from build123d import *

# Parameters (mm, degrees)
SKETCH_1_R          = 30
SKETCH_1_R_2        = 23
EXTRUDE_1_DEPTH     = 21
SKETCH_2_R          = 23
SKETCH_2_R_2        = 4.1
SKETCH_2_R_3        = 1.55
EXTRUDE_2_DEPTH     = 1
SKETCH_3_R          = 30
SKETCH_3_R_2        = 1.55
SKETCH_3_R_3        = 4.1
EXTRUDE_3_DEPTH     = 3
SKETCH_4_R          = 30
CUT_EXTRUDE_1_DEPTH = 3


with BuildPart() as part:
    # 草图1 → 凸台-拉伸1 (new body)
    with BuildSketch(Plane(origin=(0, 0, 0), x_dir=(1, 0, 0), z_dir=(0, 1, 0))):
        Circle(SKETCH_1_R)
        Circle(SKETCH_1_R_2, mode=Mode.SUBTRACT)
    extrude(amount=EXTRUDE_1_DEPTH)

    # 草图2 → 凸台-拉伸2 (add)
    with BuildSketch(Plane.XZ):
        Circle(SKETCH_2_R)
        Circle(SKETCH_2_R_2, mode=Mode.SUBTRACT)
        with Locations((6, 0)):
            Circle(SKETCH_2_R_3, mode=Mode.SUBTRACT)
        with Locations((-6, 0)):
            Circle(SKETCH_2_R_3, mode=Mode.SUBTRACT)
        with Locations((0, 6.5)):
            Circle(SKETCH_2_R_3, mode=Mode.SUBTRACT)
        with Locations((0, -6.5)):
            Circle(SKETCH_2_R_3, mode=Mode.SUBTRACT)
        with BuildLine():
            ThreePointArc((13.744660155, 13.324975875), (0.2967616, 19.141123201), (-13.324975875, 13.744660155))
            ThreePointArc((-13.324975875, 13.744660155), (-13.412668503, 8.088485652), (-7.756494001, 8.000793024))
            ThreePointArc((-7.756494001, 8.000793024), (0.172745496, 11.142084508), (8.000793024, 7.756494001))
            ThreePointArc((8.000793024, 7.756494001), (13.656967527, 7.668801373), (13.744660155, 13.324975875))
        make_face(mode=Mode.SUBTRACT)
        with BuildLine():
            ThreePointArc((13.744660155, -13.324975875), (0.2967616, -19.141123201), (-13.324975875, -13.744660155))
            ThreePointArc((-13.324975875, -13.744660155), (-13.412668503, -8.088485652), (-7.756494001, -8.000793024))
            ThreePointArc((-7.756494001, -8.000793024), (0.172745496, -11.142084508), (8.000793024, -7.756494001))
            ThreePointArc((8.000793024, -7.756494001), (13.656967527, -7.668801373), (13.744660155, -13.324975875))
        make_face(mode=Mode.SUBTRACT)
    extrude(amount=-EXTRUDE_2_DEPTH)

    # 草图3 → 凸台-拉伸3 (add)
    with BuildSketch(Plane.XZ):
        Circle(SKETCH_3_R)
        with Locations((0, -6.5)):
            Circle(SKETCH_3_R_2, mode=Mode.SUBTRACT)
        with Locations((6, 0)):
            Circle(SKETCH_3_R_2, mode=Mode.SUBTRACT)
        Circle(SKETCH_3_R_3, mode=Mode.SUBTRACT)
        with Locations((0, 6.5)):
            Circle(SKETCH_3_R_2, mode=Mode.SUBTRACT)
        with BuildLine():
            ThreePointArc((-7.756494001, -8.000793024), (-13.412668503, -8.088485652), (-13.324975875, -13.744660155))
            ThreePointArc((-13.324975875, -13.744660155), (0.2967616, -19.141123201), (13.744660155, -13.324975875))
            ThreePointArc((13.744660155, -13.324975875), (13.656967527, -7.668801373), (8.000793024, -7.756494001))
            ThreePointArc((8.000793024, -7.756494001), (0.172745496, -11.142084508), (-7.756494001, -8.000793024))
        make_face(mode=Mode.SUBTRACT)
        with BuildLine():
            ThreePointArc((8.000793024, 7.756494001), (13.656967527, 7.668801373), (13.744660155, 13.324975875))
            ThreePointArc((13.744660155, 13.324975875), (0.2967616, 19.141123201), (-13.324975875, 13.744660155))
            ThreePointArc((-13.324975875, 13.744660155), (-13.412668503, 8.088485652), (-7.756494001, 8.000793024))
            ThreePointArc((-7.756494001, 8.000793024), (0.172745496, 11.142084508), (8.000793024, 7.756494001))
        make_face(mode=Mode.SUBTRACT)
    extrude(amount=EXTRUDE_3_DEPTH)

    # 草图4 → 切除-拉伸1 (cut)
    with BuildSketch(Plane(origin=(0, 21, 0), x_dir=(1, 0, 0), z_dir=(0, 1, 0))):
        Circle(SKETCH_4_R)
    extrude(amount=-CUT_EXTRUDE_1_DEPTH, mode=Mode.SUBTRACT)


solid = part.part
Source: CAD feature listing. Evaluate the final solid. Frame: model axes, mm. A direction names the side the tool comes from. Coordinates: 2 decimals unless noted, no trailing zeros. Order: outer loops, then holes, each group sorted by start corner. A loop starts at its lowest first (then second) coordinate and runs counter-clockwise, first axis right, second up.
Item 1: Cut plane B-B (z = 0). Return loops of the section in (x, y), plus the area to 3 significant figures.
Output values:
outline: (-30, -3) - (-4.1, -3) - (-4.1, 1) - (-4.45, 1) - (-4.45, 0) - (-7.55, 0) - (-7.55, 1) - (-23, 1) - (-23, 18) - (-30, 18) - close; (4.1, -3) - (4.45, -3) - (4.45, 1) - (4.1, 1) - close; (7.55, -3) - (30, -3) - (30, 18) - (23, 18) - (23, 1) - (7.55, 1) - close
area: 430 mm2
Item 2: Cut plane A-A (x = 0). Return loops of the section in (y, z), plus the area to 3 significant figures.
Output values:
outline: (-3, -30) - (18, -30) - (18, -23) - (1, -23) - (1, -19.14) - (-3, -19.14) - close; (-3, -11.14) - (1, -11.14) - (1, -8.05) - (-3, -8.05) - close; (-3, -4.95) - (1, -4.95) - (1, -4.1) - (-3, -4.1) - close; (-3, 4.1) - (1, 4.1) - (1, 4.95) - (-3, 4.95) - close; (-3, 8.05) - (1, 8.05) - (1, 11.14) - (-3, 11.14) - close; (-3, 19.14) - (1, 19.14) - (1, 23) - (18, 23) - (18, 30) - (-3, 30) - close
area: 356 mm2
Item 3: Pull-direction query (Z, two-part tool) for faces 4 (the face through (-29.97, 7.65, 1.32)), 5 (the face through (-7, -3, 0)), 6 (the face through (-7.55, 0.49, 0.07)), 7 (the face through (0.3, -0.97, -11.14)); classes: pulls with the +Z half, pulls with the -Z half, needs draft (parallel to the pull), parting line crosses it, or undercut.
Output values:
face 4: parting line crosses it
face 5: needs draft
face 6: undercut
face 7: undercut
Item 4: Set-up query: faces 1 (the face through (-0.3, 1, -4.8)), 2 (the face through (0.086, -0.972, -19.143)), 3 (the face through (15, 18, 18)). Return all of +Z, -Z, +X, -X, +Y, -Y with unobstructed straight access to the full face (end or side cutting, diameter ignored); none if empty.
Output values:
face 1: +Y
face 2: +Y, -Y
face 3: +Z, -Z, +X, -X, +Y
Item 5: Material intervals for line 1 (Z direction, x = 0, y = -1.45); line 2 (Z direction, x = -6, y = 0.35); line 3 (Y direction, x = -17, z = 12), sorted ascending.
Output values:
line 1: z = -30 to -19.14, -11.14 to -8.05, -4.95 to -4.1, 4.1 to 4.95, 8.05 to 11.14, 19.14 to 30
line 2: z = -29.39 to -18.18, -9.39 to -1.55, 1.55 to 9.39, 18.18 to 29.39
line 3: y = -3 to 1
Item 6: First-contact query: P1, Ø1.5, axis at x = -5.5, z = 0.5, coming from the +Y side; P2, Ø23, axis at x = -10, z = -5.5, coming from the +Y side; P3, Ø10.5, axis at x = 0, z = 0, coming from the -Y side; P4, Ø1, axis at x = -16.5, y = 9.5, coming from the +Z side. Flat tips, straight axial feed; report the tip coordinate or a pass-through.
Output values:
P1: stops at y = 0
P2: stops at y = 1
P3: stops at y = -3
P4: stops at z = 25.38
Item 7: Cut plane D-D (y = 2.5). Return loops of the section in (x, z).
Output values:
outline: circle Ø60 at (0, 0); hole circle Ø46 at (0, 0)
Item 8: Cut plane C-C (x = -6). Return loops of the section in (y, z).
Output values:
outline: (-3, -29.39) - (18, -29.39) - (18, -22.2) - (1, -22.2) - (1, -18.18) - (-3, -18.18) - close; (-3, -9.39) - (1, -9.39) - (1, -1.55) - (0, -1.55) - (0, 1.55) - (1, 1.55) - (1, 9.39) - (-3, 9.39) - close; (-3, 18.18) - (1, 18.18) - (1, 22.2) - (18, 22.2) - (18, 29.39) - (-3, 29.39) - close
